Work out the finished part from the listing and answer in its coordinate system (mm). A direction names the side the tool comes from. Coordinates: 2 decimals unless noted, no trailing zeros. Order: outer loops, then holes, each group sorted by start corner. A loop starts at its lowest first (then second) coordinate and runs counter-clockwise, first axis right, second up. Notation, with made-up numbers: (32.25, 58.25) -> (64.25, 58.25) arc R13 ccw to (64.25, 63.25) -> close; hole circle Ø6 at (47.25, 26.5). An arc over 180 degrees is marked (long way). Use one line per item in the form item = value.
from build123d import *

# Parameters (mm, degrees)
SKETCH1_R                = 8
BOSS_EXTRUDE1_DEPTH      = 10
BOSS_EXTRUDE3_DEPTH      = 88
BOSS_EXTRUDE3_DEPTH_BACK = 10
SKETCH1_4_W              = 38
SKETCH1_4_H              = 10
BOSS_EXTRUDE4_START      = 88
BOSS_EXTRUDE4_DEPTH      = 10
BOSS_EXTRUDE5_START      = 100
SKETCH1_6_R              = 19
SKETCH1_6_R_2            = 2
SKETCH1_6_R_3            = 8
BOSS_EXTRUDE5_DEPTH      = 25
SKETCH1_7_W              = 31
SKETCH1_7_H              = 10
BOSS_EXTRUDE6_DEPTH      = 10
FILLET1_R                = 31
FILLET3_R                = 5
FILLET4_R                = 15
BOSS_EXTRUDE7_START      = -24
BOSS_EXTRUDE7_DEPTH      = 10
FILLET5_R                = 20


with BuildPart() as part:
    # Sketch1 → Boss-Extrude1 (new body)
    with BuildSketch(Plane.XY):
        Polygon((-38, 10), (0, 10), (0, 45), (-69, 45), (-69, 10), align=None)
        with Locations((-47, 27)):
            Circle(SKETCH1_R, mode=Mode.SUBTRACT)
    extrude(amount=-BOSS_EXTRUDE1_DEPTH)

    # Sketch1<4> → Boss-Extrude3 (add, two sides: drawn at the far end of the back side and taken through both)
    with BuildSketch(Plane.XY.offset(-BOSS_EXTRUDE3_DEPTH_BACK)):
        with Locations((-19, 5)):
            Rectangle(SKETCH1_4_W, SKETCH1_4_H)
    extrude(amount=BOSS_EXTRUDE3_DEPTH + BOSS_EXTRUDE3_DEPTH_BACK)

    # Sketch1<5> → Boss-Extrude4 (add)
    with BuildSketch(Plane.XY.offset(BOSS_EXTRUDE4_START)):
        with BuildLine():
            Line((0, -30), (0, 0))
            Line((0, 0), (-38, 0))
            Line((-38, 0), (-38, -30))
            ThreePointArc((-38, -30), (-19, -11), (0, -30))
        make_face()
    extrude(amount=-BOSS_EXTRUDE4_DEPTH)

    # Sketch1<6> → Boss-Extrude5 (add)
    with BuildSketch(Plane.XY.offset(BOSS_EXTRUDE5_START)):
        with Locations((-19, -30)):
            Circle(SKETCH1_6_R)
        with Locations((-22.235238064, -17.925927171)):
            Circle(SKETCH1_6_R_2, mode=Mode.SUBTRACT)
        with Locations((-31.074072829, -26.764761936)):
            Circle(SKETCH1_6_R_2, mode=Mode.SUBTRACT)
        with Locations((-27.838834765, -38.838834765)):
            Circle(SKETCH1_6_R_2, mode=Mode.SUBTRACT)
        with Locations((-15.764761936, -42.074072829)):
            Circle(SKETCH1_6_R_2, mode=Mode.SUBTRACT)
        with Locations((-6.925927171, -33.235238064)):
            Circle(SKETCH1_6_R_2, mode=Mode.SUBTRACT)
        with Locations((-10.161165235, -21.161165235)):
            Circle(SKETCH1_6_R_2, mode=Mode.SUBTRACT)
        with Locations((-19, -30)):
            Circle(SKETCH1_6_R_3, mode=Mode.SUBTRACT)
    extrude(amount=-BOSS_EXTRUDE5_DEPTH)

    # Sketch1<7> → Boss-Extrude6 (add)
    with BuildSketch(Plane.XY):
        with Locations((-53.5, 5)):
            Rectangle(SKETCH1_7_W, SKETCH1_7_H)
    extrude(amount=-BOSS_EXTRUDE6_DEPTH)

    # Fillet1
    fillet1_edges = [part.edges().sort_by_distance(p)[0] for p in [
        (-38, 5, 0),
    ]]
    fillet(fillet1_edges, radius=FILLET1_R - 0.0001)  # a hair under: the kernel refuses the full size

    # Fillet3
    fillet3_edges = [part.edges().sort_by_distance(p)[0] for p in [
        (-19, 0, 78),
    ]]
    fillet(fillet3_edges, radius=FILLET3_R)

    # Fillet4
    fillet4_edges = [part.edges().sort_by_distance(p)[0] for p in [
        (-19, 10, 88),
    ]]
    fillet(fillet4_edges, radius=FILLET4_R)

    # Sketch2 → Boss-Extrude7 (add)
    with BuildSketch(Plane(origin=(0, 0, 0), x_dir=(0, 0, -1), z_dir=(1, 0, 0)).offset(BOSS_EXTRUDE7_START)):
        with BuildLine():
            Line((-98, -13), (-88, -13))
            Line((-88, -13), (-88, -5))
            ThreePointArc((-88, -5), (-83.606601718, 5.606601718), (-73, 10))
            Line((-73, 10), (0, 10))
            Line((0, 10), (0, 20))
            Line((0, 20), (-73, 20))
            ThreePointArc((-73, 20), (-90.67766953, 12.67766953), (-98, -5))
            Line((-98, -5), (-98, -13))
        make_face()
    extrude(amount=BOSS_EXTRUDE7_DEPTH)

    # Fillet5
    fillet5_edges = [part.edges().sort_by_distance(p)[0] for p in [
        (-19, 20, 0),
    ]]
    fillet(fillet5_edges, radius=FILLET5_R)


solid = part.part
(1) Section D-D on z = 16 is taken. Write down the section's boundary in (x, y), plus the area to 3 significant figures.
Data:
outline = (-41.87, 0) -> (0, 0) -> (0, 10) -> (-14, 10) -> (-14, 20.4) -> (-24, 20.4) -> (-24, 10) -> (-41.87, 10) -> close
area = 523 mm²
(2) Section A-A on x = -47 is taken. Write down the section's boundary in (y, z).
Data:
outline = (0, -10) -> (19, -10) -> (19, 0) -> (10, 0) -> (10, 9.16) -> (0, 9.16) -> close; (35, -10) -> (45, -10) -> (45, 0) -> (35, 0) -> close
(3) Section B-B on y = 27 is taken. Write down the section's boundary in (x, z).
Data:
outline = (-69, -10) -> (-55, -10) -> (-55, 0) -> (-69, 0) -> close; (-39, -10) -> (0, -10) -> (0, 0) -> (-14, 0) -> (-14, 4.8) -> (-24, 4.8) -> (-24, 0) -> (-39, 0) -> close
(4) Straight lines are drawn through the part: line 1 along Y through (x, z) = (-7, 76); line 2 along Z through (x, y) = (-49, 18.5); line 3 along Y through (x, z) = (-21, 40.5). For each, find the intervals that lie inside material, in ascending order.
Data:
line_1 = -44.73 to -35.23, -31.24 to -15.27, -1 to 9.7
line_2 = -10 to 0
line_3 = 0 to 20
(5) Which of the six approach directions +Z, -Z, +X, -X, +Y, -Y give full straight-line access (tool end or side, diameter ignored) to faces 4 (the flat face through (-32, 10, 36)), 5 (the flat face through (-14, 12, 49)), 6 (the flat face through (-19.3, -38.2, 75))?
Data:
face_4 = +Z, -X, +Y
face_5 = +Z, +X, +Y
face_6 = -Z, +X, -X, -Y
(6) Each of these flat-tipped pins is pushed along its axis until it touches: P1, Ø15.5, axis at y = 13, z = 29, coming from the -X side; P2, Ø7.5, axis at x = -27.5, y = -19.5, coming from the -Z side; P3, Ø1, axis at x = -54, y = 9, coming from the +Z side. Where does it stop, or does it pass through?
Data:
P1 = -39.38
P2 = 75
P3 = 4.15
(7) The mould has two halves that part along X. Classify faces 1 (the cylindrical face through (-28.099, -36.856, 87.675)), 2 (the flat face through (0, 5, 36)), 3 (the flat face through (-19, 20, 46)): released by +X, released by -X, zero draft, split by the parting line, or undercut.
Data:
face_1 = undercut
face_2 = released by +X
face_3 = zero draft
